Geometry: see drawing. Coordinates: mm, zero at the bounding-box minimum. Round coordinates to 2 decimals unless told otherwise and drop trailing zeros. Loops run counter-clockwise (first coordinate to the right, second up) from the corner with the lowest first, then second, coordinate; pieces in that order, holes last. Notation, with made-up numbers: (2.5, 66.25) - (20.5, 66.25) arc R29 ccw to (20.5, 103.25) - close; hole circle Ø8 at (-10, -16.5). An arc over 180 degrees is marked (long way). Write item = value, one per line. Start each with the question number.
Item 1: Section C-C (x = 6.25). Return loops of the section in (y, z), plus the area to 3 significant figures.
Item 2: Section B-B (z = 12.5). Return loops of the section in (x, y), plus the area to 3 significant figures.
Item 3: Draft query along X for the marked faces 1 and 2. Return one class per face: pulls with the +X half, pulls with the -X half, needs draft (parallel to the pull), parting line crosses it, or undercut.
Item 4: Section A-A (x = 12.5). Return loops of the section in (y, z).
Item 5: First-contact query: pin 1 (1 mm diameter, centred on x = 3, z = 9, fed in from +Y); pin 2 (1 mm diameter, centred on y = 36.5, z = 7.5, fed in from -X); pin 3 (8 mm diameter, centred on x = 19.5, z = 8.5, fed in from +Y). Flat tips, straight axial feed; report the tip coordinate or a pass-through.
Item 6: Section D-D (z = 5). Return loops of the section in (x, y), plus the area to 3 significant figures.
Item 7: Line query: line 1 (Z direction, x = 12, y = 8); line 2 (X direction, y = 21, z = 12.5); line 3 (Z direction, x = 7.25, y = 5). Output: solid intervals per line, ascending. Write a range as from..to.
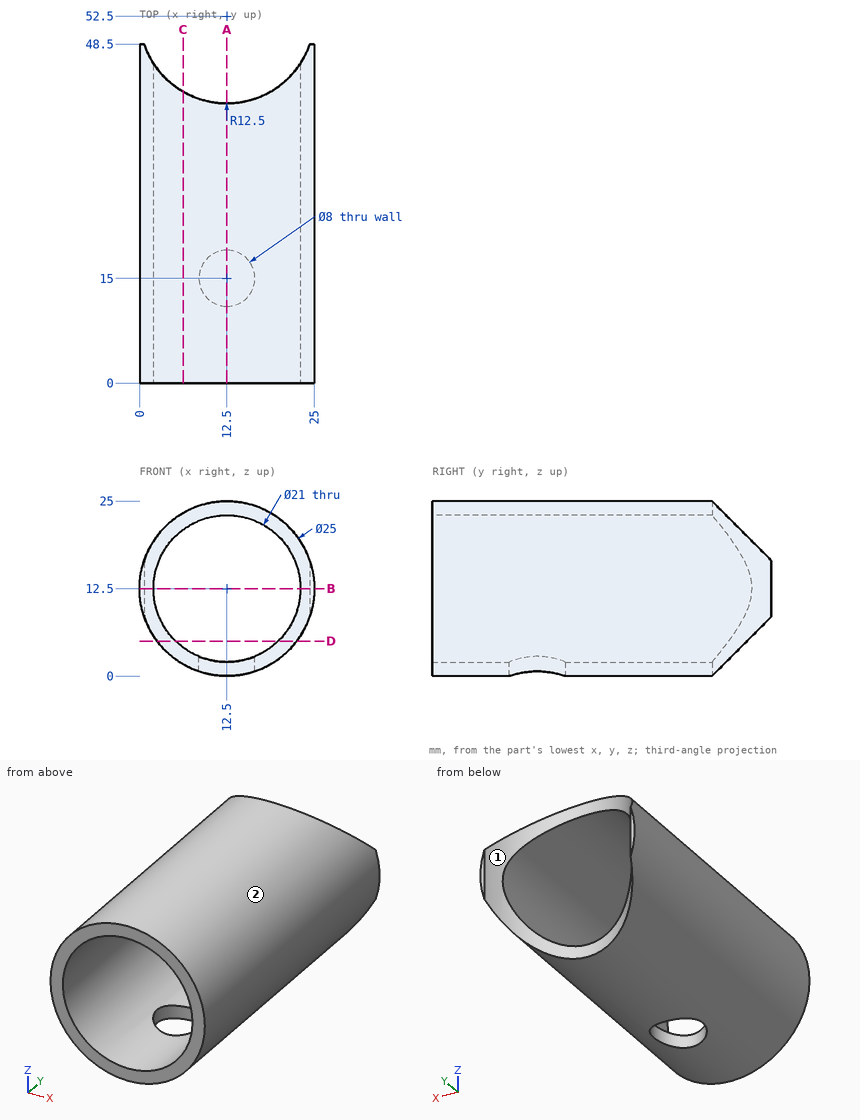
Taken from the geometry:
q1.outline = (0, 1.67) - (41.67, 1.67) - (41.67, 4.06) - (0, 4.06) - close; (0, 20.94) - (41.67, 20.94) - (41.67, 23.33) - (0, 23.33) - close
q1.area = 199 mm^2
q2.outline = (0, 0) - (2, 0) - (2, 45.72) arc R12.5 cw to (0.66, 48.5) - (0, 48.5) - close; (23, 0) - (25, 0) - (25, 48.5) - (24.34, 48.5) arc R12.5 cw to (23, 45.72) - close
q2.area = 190 mm^2
q3.face_1 = undercut
q3.face_2 = parting line crosses it
q4.outline = (0, 0) - (11, 0) - (11, 2) - (0, 2) - close; (0, 23) - (40, 23) - (40, 25) - (0, 25) - close; (19, 0) - (40, 0) - (40, 2) - (19, 2) - close
q5.pin_1 = 45
q5.pin_2 = 0.84
q5.pin_3 = 46.56
q6.outline = (2.5, 0) - (5.15, 0) - (5.15, 42.39) arc R12.5 cw to (2.5, 45) - close; (19.85, 0) - (22.5, 0) - (22.5, 45) arc R12.5 cw to (19.85, 42.39) - close
q6.area = 231 mm^2
q7.line_1 = 0.01..2.01, 22.99..24.99
q7.line_2 = 0..2, 23..25
q7.line_3 = 1.16..3.41, 21.59..23.84
